Verification items for the finished model (mm, model axes). A direction names the side the tool comes from. Coordinates: 2 decimals unless noted, no trailing zeros. Write each loop counter-clockwise with the first axis right and the second up, starting at its lowest first coordinate (ties: lowest second). Pieces come first, ordered by that corner, then holes. Notation, with made-up numbers: (49, -0.75) -> (59, -0.75) arc R10 ccw to (59, 6.25) -> close; hole circle Ø2 at (-39.75, 0). An arc over 180 degrees is marked (long way). Answer in a Markdown table with one row per item.
```python
from build123d import *

# Parameters (mm, degrees)
SKETCH1_W           = 76.2
SKETCH1_H           = 88.9
SKETCH1_H_2         = 57.15
SKETCH1_W_2         = 38.1
BOSS_EXTRUDE1_DEPTH = 76.2


with BuildPart() as part:
    # Sketch1 → Boss-Extrude1 (new body)
    with BuildSketch(Plane(origin=(0, 0, 0), x_dir=(1, 0, 0), z_dir=(0, 1, 0))):
        Rectangle(SKETCH1_W, SKETCH1_H)
        with Locations((0, 73.025)):
            Rectangle(SKETCH1_W, SKETCH1_H_2)
        with Locations((57.15, 0)):
            Rectangle(SKETCH1_W_2, SKETCH1_H)
        with Locations((0, -73.025)):
            Rectangle(SKETCH1_W, SKETCH1_H_2)
        with Locations((-57.15, 0)):
            Rectangle(SKETCH1_W_2, SKETCH1_H)
    extrude(amount=BOSS_EXTRUDE1_DEPTH)


solid = part.part
```
1. Sectioned sample at A-A, the plane y = 59. Record the cut outline in (x, z), and give its area (3 significant figures).
Findings below:
| item | result |
|---|---|
| outline | (-76.2, -44.45) -> (-38.1, -44.45) -> (-38.1, -101.6) -> (38.1, -101.6) -> (38.1, -44.45) -> (76.2, -44.45) -> (76.2, 44.45) -> (38.1, 44.45) -> (38.1, 101.6) -> (-38.1, 101.6) -> (-38.1, 44.45) -> (-76.2, 44.45) -> close |
| area | 22,300 mm² |
2. Material ranges on probe 1 along Z at (x, y) = (-59.5, 66.5); probe 2 along X at (y, z) = (19, -53), recorded low to high. Write a range as from..to.
Findings below:
| item | result |
|---|---|
| probe 1 | z = -44.45..44.45 |
| probe 2 | x = -38.1..38.1 |
3. Sectioned sample at C-C, the plane x = -61.5. Record the cut outline in (y, z).
Findings below:
| item | result |
|---|---|
| outline | (0, -44.45) -> (76.2, -44.45) -> (76.2, 44.45) -> (0, 44.45) -> close |
4. Sectioned sample at B-B, the plane z = 54. Record the cut outline in (x, y), and give its area (3 significant figures).
Findings below:
| item | result |
|---|---|
| outline | (-38.1, 0) -> (38.1, 0) -> (38.1, 76.2) -> (-38.1, 76.2) -> close |
| area | 5,810 mm² |
5. Go/stop test with flat-tipped pins: pin 1 (19 mm diameter, centred on x = 66.5, y = 23, fed in from -Z); pin 2 (17 mm diameter, centred on y = 43, z = 79.5, fed in from -X); pin 3 (19 mm diameter, centred on x = 65, y = 22, fed in from +Z). Record where each tip stops, or that it passes through.
Findings below:
| item | result |
|---|---|
| pin 1 | stops at z = -44.45 |
| pin 2 | stops at x = -38.1 |
| pin 3 | stops at z = 44.45 |
6. Access from +Z, -Z, +X, -X, +Y, -Y to the whole of each face (thin tool, end or side, straight path). Record for faces 1 (the face through (-57, 38, 44.45)), 2 (the face through (38.1, 38, 73)), 3 (the face through (-38.1, 38, -73)), 4 (the face through (57, 38, -44.45)).
Findings below:
| item | result |
|---|---|
| face 1 | +Z, -X, +Y, -Y |
| face 2 | +Z, +X, +Y, -Y |
| face 3 | -Z, -X, +Y, -Y |
| face 4 | -Z, +X, +Y, -Y |
